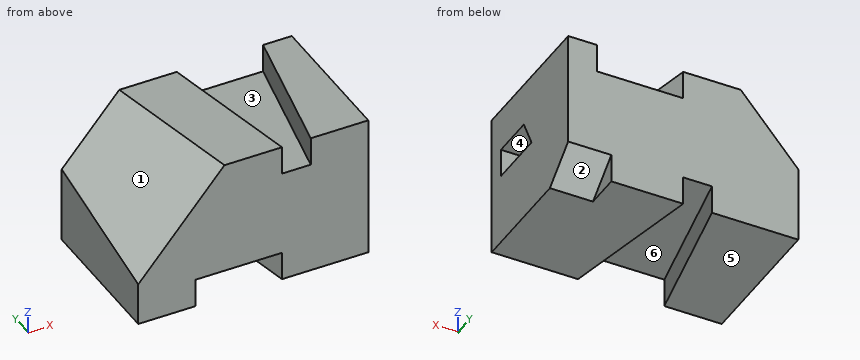
from build123d import *

# Parameters (mm, degrees)
F0_W      = 80
F0_H      = 50
F1_DEPTH  = 50
F6_DEPTH  = 10
F8_DEPTH  = 15
F10_DEPTH = 25
F12_DEPTH = 10


with BuildPart() as f1:
    # F0 (on Top) → F1 (new body)
    with BuildSketch(Plane.XY):
        with Locations((40, 25)):
            Rectangle(F0_W, F0_H)
    extrude(amount=F1_DEPTH)

    # F4: sweep along a path in F3
    with BuildLine(Plane.XY.offset(50)) as f4_path:
        Line((30, 0), (20, 50))
    # F2 (on face) → F4 (sweep, cut)
    with BuildSketch(Plane.XZ):
        Polygon((0, 50), (0, 15), (30, 50), align=None)
    sweep(path=f4_path.line, mode=Mode.SUBTRACT)

    # F5 (on face) → F6 (cut)
    with BuildSketch(Plane(origin=(0, 0, 0), x_dir=(1, 0, 0), z_dir=(0, 0, -1))):
        Polygon((50, 0), (20, 0), (30, -50), (40, -50), align=None)
    extrude(amount=-F6_DEPTH, mode=Mode.SUBTRACT)

    # F7 (on face) → F8 (cut)
    with BuildSketch(Plane.YZ.offset(80)):
        Polygon((38, 0), (50, 0), (50, 10), align=None)
    extrude(amount=-F8_DEPTH, mode=Mode.SUBTRACT)

    # F9 (on face) → F10 (cut)
    with BuildSketch(Plane.YZ.offset(80)):
        Polygon((21, 35), (6, 35), (6, 25), (26, 25), align=None)
    extrude(amount=-F10_DEPTH, mode=Mode.SUBTRACT)

    # F11 (on face) → F12 (cut)
    with BuildSketch(Plane.XY.offset(50)):
        Polygon((40, 50), (50, 0), (60, 0), (70, 50), align=None)
    extrude(amount=-F12_DEPTH, mode=Mode.SUBTRACT)


solid = f1.part
Could you check a few things on this model? Use its own coordinates, in mm. Face numbers are marked on the shaded views. A direction names the side the tool comes from. Give positions to 0.01 mm unless a question says otherwise; leave off trailing zeros. Write each loop counter-clockwise with the first axis right and the second up, starting at its lowest first coordinate (ties: lowest second). Pieces come first, ordered by that corner, then holes. Notation, with made-up numbers: (52.25, 42.5) -> (68.25, 42.5) arc R18 cw to (68.25, 73.5) -> close; hole circle Ø3 at (36.5, -30). An arc over 180 degrees is marked (long way). Answer as CSV lines item,"result". Start each with the question number.
(1) If we mould it in two halves opening along Y, with no side actions, what happens to the marked faces 1, 2, 3 and 4? For each: +Y half, -Y half, draft (parallel to the pull), parting line (faces both ways), or undercut.
(2) Which directions (+Z, -Z, +X, -X, +Y, -Y) give clear straight access to the entire face, cutting with the end or side of a thin tool? Please do the marked faces 5 and 6.
(3) I'm going to push a flat-ended pin straight in: pin 1 Ø15 at (x, y) = (52.5, 30) entering from +Z. Where does the tip first touch, or does it pass through?
(4) If we section it at D-D, the plane y = 36.5: Write out the boundary of the cut face in (x, z), and give its area (3 significant figures).
(5) If we section it at A-A, the plane x = 75: Write out the boundary of the cut face in (y, z).
(6) If we section it at C-C, the plane x = 21: Write out the boundary of the cut face in (y, z), and give its area (3 significant figures).
(7) Please list where these lines run through material, in increasing order: line 1 (X direction, y = 11, z = 42); line 2 (Z direction, x = 52, y = 10.5); line 3 (X direction, y = 44, z = 43.5).
(8) If we section it at B-B, the plane y = 27: Write out the boundary of the cut face in (x, z).
Answer list:
1,face 1,"-Y half"
1,face 2,"+Y half"
1,face 3,"draft"
1,face 4,"undercut"
2,face 5,"-Z, +X, -X, +Y, -Y"
2,face 6,"-Z, -Y"
3,pin 1,"z = 40"
4,outline,"(0, 0) -> (27.3, 0) -> (27.3, 10) -> (42.7, 10) -> (42.7, 0) -> (80, 0) -> (80, 50) -> (67.3, 50) -> (67.3, 40) -> (42.7, 40) -> (42.7, 50) -> (22.7, 50) -> (0, 23.52) -> close"
4,area,"3,300 mm^2"
5,outline,"(0, 0) -> (38, 0) -> (50, 10) -> (50, 50) -> (0, 50) -> close; hole (6, 25) -> (26, 25) -> (21, 35) -> (6, 35) -> close"
6,outline,"(0, 10) -> (5, 10) -> (5, 0) -> (50, 0) -> (50, 50) -> (45, 50) -> (0, 39.5) -> close"
6,area,"2,210 mm^2"
7,line 1,"20.94 to 47.8, 62.2 to 80"
7,line 2,"0 to 40"
7,line 3,"15.63 to 41.2, 68.8 to 80"
8,outline,"(0, 0) -> (25.4, 0) -> (25.4, 10) -> (44.6, 10) -> (44.6, 0) -> (80, 0) -> (80, 50) -> (65.4, 50) -> (65.4, 40) -> (44.6, 40) -> (44.6, 50) -> (24.6, 50) -> (0, 21.3) -> close"
